from build123d import *

# Parameters (mm, degrees)
EXTRUDE_1_DEPTH     = 3
SKETCH_2_R          = 1.6
CUT_EXTRUDE_1_DEPTH = 3
SKETCH_3_R          = 1.5
CUT_EXTRUDE_2_DEPTH = 10


with BuildPart() as part:
    # 草图1 → 凸台-拉伸1 (new body)
    with BuildSketch(Plane(origin=(0, 0, 0), x_dir=(1, 0, 0), z_dir=(0, 1, 0))):
        with BuildLine():
            Line((30, 176.457513111), (30, 103.440804328))
            ThreePointArc((30, 103.440804328), (32.320198134, 55.328281895), (39.259259259, 7.662281802))
            ThreePointArc((39.259259259, 7.662281802), (0, -40), (-39.259259259, 7.662281802))
            ThreePointArc((-39.259259259, 7.662281802), (-32.320198134, 55.328281895), (-30, 103.440804328))
            Line((-30, 103.440804328), (-30, 176.457513111))
            ThreePointArc((-30, 176.457513111), (0, 206.457513111), (30, 176.457513111))
        make_face()
    extrude(amount=EXTRUDE_1_DEPTH)

    # 草图2 → 切除-拉伸1 (cut)
    with BuildSketch(Plane(origin=(0, 3, 0), x_dir=(1, 0, 0), z_dir=(0, 1, 0))):
        with Locations(Location((0, -34.5, 0), (0, 0, 270))):
            Circle(SKETCH_2_R)
        with Locations(Location((33.842463041, 6.730809037, 0), (0, 0, 270))):
            Circle(SKETCH_2_R)
        with Locations(Location((24.500054413, 103.453580765, 0), (0, 0, 270))):
            Circle(SKETCH_2_R)
        with Locations(Location((24.500043559, 176.468944491, 0), (0, 0, 270))):
            Circle(SKETCH_2_R)
        with Locations(Location((-24.500043559, 176.468944491, 0), (0, 0, 90))):
            Circle(SKETCH_2_R)
        with Locations(Location((-24.500054413, 103.453580765, 0), (0, 0, 90))):
            Circle(SKETCH_2_R)
        with Locations(Location((-33.842463041, 6.730809037, 0), (0, 0, 90))):
            Circle(SKETCH_2_R)
    extrude(amount=-CUT_EXTRUDE_1_DEPTH, mode=Mode.SUBTRACT)

    # 草图3 → 切除-拉伸2 (cut)
    with BuildSketch(Plane(origin=(0, 3, 0), x_dir=(1, 0, 0), z_dir=(0, 1, 0))):
        with Locations(Location((0, 144.457513111, 0), (0, 0, 270))):
            Circle(SKETCH_3_R)
    extrude(amount=-CUT_EXTRUDE_2_DEPTH, mode=Mode.SUBTRACT)


solid = part.part
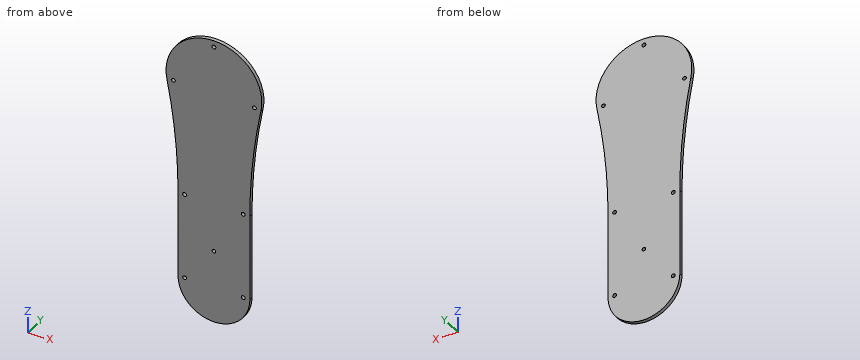
Geometry: final body of the model. Coordinates: model frame, mm. Round coordinates to 2 decimals unless told otherwise and drop trailing zeros. Loops run counter-clockwise (first coordinate to the right, second up) from the corner with the lowest first, then second, coordinate; pieces in that order, holes last. Notation, with made-up numbers: M -31,-37 L 18,-37 A34 cw 18,-4 Z; hole C -34.75,2 d4. An arc over 180 degrees is marked long. One line per question, with ' | ' between items.
(1) Material intervals for line 1 along X through (y, z) = (0.9, -6.5); line 2 along X through (y, z) = (2.15, -124.5); line 3 along X through (y, z) = (1.55, -56), sorted ascending. Write a range as from..to.
Check result:
line 1: x = -39.47..-35.43, -32.26..32.26, 35.43..39.47 | line 2: x = -30..30 | line 3: x = -32.26..32.26
(2) Cut plane A-A on y = 1.4. Give the number of separate pieces and of enclosed holes in the cut face, plus the area to 3 significant figures.
Check result:
separate pieces: 1 | enclosed holes: 8 | area: 15,200 mm2
(3) Contact query for flat-ended pins moving along their axis: P1, Ø1.5, axis at x = -23.5, y = 1, coming from the -Z side; P2, Ø1.5, axis at y = 2.5, z = -34, coming from the -X side; P3, Ø1.5, axis at x = 27, y = 1, coming from the +Z side. Output: stop coordinate, or through.
Check result:
P1: stops at z = -196.01 | P2: stops at x = -34.95 | P3: stops at z = 30.18
(4) Cut plane B-B on z = -131.5. Return the cut outline in (x, y), plus the area to 3 significant figures.
Check result:
outline: M -30,0 L 30,0 L 30,3 L -30,3 Z | area: 180 mm2
(5) Cut plane C-C on z = 16. Return the cut outline in (x, y).
Check result:
outline: M -36.66,0 L 36.66,0 L 36.66,3 L -36.66,3 Z
